Autodesk Inventor part; units mm, degrees
ref_plane "YZ Plane" through (0, 0, 0) normal (1, 0, 0) x (0, 1, 0)
ref_plane "XZ Plane" through (0, 0, 0) normal (0, 1, 0) x (-1, 0, 0)
ref_plane "XY Plane" through (0, 0, 0) normal (0, 0, 1) x (1, 0, 0)
sketch "Sketch1" plane through (0, 0, 0) normal (0, 1, 0) x (-1, 0, 0)
  circle A0 centre (0, 0) radius 1.5
  dimension "d0" = 3
extrude "Extrusion1" add sketch "Sketch1" against normal blind 8
sketch "Sketch2" plane through (0, 0, 0) normal (0, 1, 0) x (1, 0, 0)
  line L0 (-14.5, -6) -> (3.5, -6)
  line L1 (3.5, -6) -> (3.5, 6)
  line L2 (3.5, 6) -> (-14.5, 6)
  line L3 (-14.5, 6) -> (-14.5, -6)
  line L4 (-14.5, -6) -> (3.5, 6) construction
  line L5 (3.5, -6) -> (-14.5, 6) construction
  point P0 (0, 0)
  point P1 (-5.5, 0)
  point P2 (-5.5, 0)
  dimension "d3" = 18
  dimension "d4" = 12
  dimension "d5" = 3.5
extrude "Extrusion2" add sketch "Sketch2" along normal blind 10
sketch "Sketch3" plane through (-14.5, 0, -6) normal (-1, 0, 0) x (0, 0, 1)
  line L0 (0, 0) -> (12, 0)
  line L1 (12, 0) -> (12, 10)
  line L2 (0, 10) -> (12, 10)
  line L3 (0, 0) -> (0, 10)
  circle A0 centre (6, 5) radius 5
  point P0 (6, 0)
  point P1 (0, 5)
  point P2 (6, 10)
  dimension "d8" = 10
extrude "Extrusion3" add sketch "Sketch3" along normal blind 10.6 contours A0
fillet "Fillet1" radius 1 2 edges at (3.5, 5, -6) (3.5, 5, 6)
sketch "Sketch4" plane through (0, 10, 0) normal (0, 1, 0) x (1, 0, 0)
  line L0 (2.5, 6) -> (-14.5, 6)
  line L1 (-14.5, -6) -> (2.5, -6)
  line L2 (3.5, -5) -> (3.5, 5)
  point P0 (0, 0)
  point P1 (2, 4.5)
  point P2 (2, -4.5)
  dimension "d12" = 1.5
  dimension "d13" = 1.5
  dimension "d14" = 1.5
hole "Hole1" at (2, 10, -4.5) at (2, 10, 4.5) direction (0, -1, 0) diameter 2 end through all
properties part number "MotorRightAngle"
Verification items for the finished model (mm, model axes). A direction names the side the tool comes from. Give positions to 0.01 mm unless a question says otherwise; leave off trailing zeros. Loops run counter-clockwise (first coordinate to the right, second up) from the corner with the lowest first, then second, coordinate; pieces in that order, holes last.
1) Set-up check for faces 1 (the flat face through (-14.5, 5.7, 5.2)), 2 (the flat face through (-14.5, 5, -5.2)), 3 (the flat face through (-6, 5, 6)), 4 (the cylindrical face through (-20, 8, -4)): record each of +Z, -Z, +X, -X, +Y, -Y from which the full face is reachable in a straight line by a thin tool's end or side.
2) Depth check by flat-ended pin: pin 1 Ø8 at (x, y) = (-21, 2) entering from +Z; pin 2 Ø3 at (x, z) = (2, -4.5) entering from -Y. Enter the tip coordinate at first touch or a pass-through.
3) Draft check along X on faces 5 (the cylindrical face through (2.6, 4.9, 3.7)), 6 (the flat face through (-6, 10, 0)), 7 (the cylindrical face through (1.5, -3.94, 0.07)). Enter one of: pulls with the +X half, pulls with the -X half, needs draft (parallel to the pull), parting line crosses it, or undercut.
4) Sectioned sample at D-D, the plane z = -4.5. Enter the section's corners in (x, y), then the cut area to 3 significant figures.
5) Thickness scan on line 1 along Z through (x, y) = (2, 4); line 2 along X through (y, z) = (5, 4.5); line 3 along X through (y, z) = (2.5, 4.5). Record the ranges inside material, lowest first.
6) Sectioned sample at A-A, the plane y = 2. Enter the section's corners in (x, z).
7) Sectioned sample at C-C, the plane z = 3. Enter the section's corners in (x, y).
8) Sectioned sample at B-B, the plane x = 2. Enter the section's corners in (y, z).
Answers:
1. face 1: +Z, -X
1. face 2: -Z, -X
1. face 3: +Z, +X, -X, +Y, -Y
1. face 4: -X
2. pin 1: stops at z = 5
2. pin 2: stops at y = 0
3. face 5: undercut
3. face 6: needs draft
3. face 7: parting line crosses it
4. outline: (-25.1, 2.82) - (-14.5, 2.82) - (-14.5, 0) - (1, 0) - (1, 10) - (-14.5, 10) - (-14.5, 7.18) - (-25.1, 7.18) - close; (3, 0) - (3.5, 0) - (3.5, 10) - (3, 10) - close
4. area: 206 mm2
5. line 1: z = -6 to -5.5, -3.5 to 3.5, 5.5 to 6
5. line 2: x = -25.1 to 1, 3 to 3.5
5. line 3: x = -14.5 to 1, 3 to 3.5
6. outline: (-25.1, -4) - (-14.5, -4) - (-14.5, -6) - (2.5, -6) arc R1 ccw to (3.5, -5) - (3.5, 5) arc R1 ccw to (2.5, 6) - (-14.5, 6) - (-14.5, 4) - (-25.1, 4) - close; hole circle Ø2 at (2, -4.5); hole circle Ø2 at (2, 4.5)
7. outline: (-25.1, 1) - (-14.5, 1) - (-14.5, 0) - (3.5, 0) - (3.5, 10) - (-14.5, 10) - (-14.5, 9) - (-25.1, 9) - close
8. outline: (0, -6) - (10, -6) - (10, -5.5) - (0, -5.5) - close; (0, -3.5) - (10, -3.5) - (10, 3.5) - (0, 3.5) - close; (0, 5.5) - (10, 5.5) - (10, 6) - (0, 6) - close
